Check sheet for the modelled part. Datum: model origin and axes. Units: mm. Face numbers are marked on the shaded views. A direction names the side the tool comes from. Give positions to 0.01 mm unless a question says otherwise; leave off trailing zeros. Order: outer loops, then holes, each group sorted by start corner. A loop starts at its lowest first (then second) coordinate and runs counter-clockwise, first axis right, second up.
```python
from build123d import *
from OCP.BRepFilletAPI import BRepFilletAPI_MakeChamfer

# Parameters (mm, degrees)
SKETCH1_W                                       = 42.2
SKETCH1_H                                       = 42.2
SKETCH1_R                                       = 12.5
SKETCH1_R_2                                     = 2
BOSS_EXTRUDE1_DEPTH                             = 2
SKETCH2_W                                       = 42.2
SKETCH2_H                                       = 20
SKETCH2_R                                       = 1.625
BOSS_EXTRUDE2_DEPTH                             = 5
BOSS_EXTRUDE3_DEPTH                             = 3.5
BOSS_EXTRUDE3_DEPTH_BACK                        = 2
SKETCH3_W                                       = 8.75
SKETCH3_H                                       = 23.25
SKETCH3_W_2                                     = 2.5
SKETCH3_H_2                                     = 7
CUT_EXTRUDE1_START                              = -3.5
SKETCH4_W                                       = 4.5
SKETCH4_H                                       = 7
CUT_EXTRUDE1_DEPTH                              = 3.5
CSK_FOR_M3_FLAT_HEAD_MACHINE_SCREW1_D           = 3.4
CSK_FOR_M3_FLAT_HEAD_MACHINE_SCREW1_CSINK_D     = 6.5
CSK_FOR_M3_FLAT_HEAD_MACHINE_SCREW1_CSINK_ANGLE = 90
SKETCH10_W                                      = 8.75
SKETCH10_H                                      = 23.25
SKETCH10_W_2                                    = 2.5
SKETCH10_H_2                                    = 7
BOSS_EXTRUDE4_DEPTH                             = 4
CUT_EXTRUDE3_DEPTH                              = 10
CHAMFER1_SIZE                                   = 10
FILLET2_R                                       = 3
FILLET3_R                                       = 3
FILLET4_R                                       = 3
CHAMFER2_SIZE                                   = 1
CHAMFER2_SIZE2                                  = 0.707106781
CHAMFER3_SIZE                                   = 0.5


with BuildPart() as part:
    # Sketch1 → Boss-Extrude1 (new, symmetric)
    with BuildSketch(Plane.XY.offset(1.5)):
        Rectangle(SKETCH1_W, SKETCH1_H)
        Circle(SKETCH1_R, mode=Mode.SUBTRACT)
        with Locations((15.5, 15.5)):
            Circle(SKETCH1_R_2, mode=Mode.SUBTRACT)
        with Locations((15.5, -15.5)):
            Circle(SKETCH1_R_2, mode=Mode.SUBTRACT)
        with Locations((-15.5, -15.5)):
            Circle(SKETCH1_R_2, mode=Mode.SUBTRACT)
        with Locations((-15.5, 15.5)):
            Circle(SKETCH1_R_2, mode=Mode.SUBTRACT)
    extrude(amount=BOSS_EXTRUDE1_DEPTH, both=True)

    # Sketch2 → Boss-Extrude2 (add)
    with BuildSketch(Plane.XZ.offset(21.1)):
        Rectangle(SKETCH2_W, SKETCH2_H)
        with Locations(Location((8, 7.5, 0), (0, 0, 270))):
            Circle(SKETCH2_R, mode=Mode.SUBTRACT)
        with Locations(Location((8, -7.5, 0), (0, 0, 270))):
            Circle(SKETCH2_R, mode=Mode.SUBTRACT)
        with Locations(Location((-8, -7.5, 0), (0, 0, 270))):
            Circle(SKETCH2_R, mode=Mode.SUBTRACT)
        with Locations(Location((-8, 7.5, 0), (0, 0, 270))):
            Circle(SKETCH2_R, mode=Mode.SUBTRACT)
    extrude(amount=BOSS_EXTRUDE2_DEPTH)

    # Sketch3 → Boss-Extrude3 (add, two sides: drawn at the far end of the back side and taken through both)
    # profile 1 of 2: a face of its own
    with BuildSketch(Plane.XY.offset(-BOSS_EXTRUDE3_DEPTH_BACK)):
        with Locations((-25.475, -14.475)):
            Rectangle(SKETCH3_W, SKETCH3_H)
        with Locations((-24.1, -9.1)):
            Rectangle(SKETCH3_W_2, SKETCH3_H_2, mode=Mode.SUBTRACT)
        with Locations((-24.1, -19.85)):
            Rectangle(SKETCH3_W_2, SKETCH3_H_2, mode=Mode.SUBTRACT)
    # profile 2 of 2: a face of its own
    with BuildSketch(Plane.XY.offset(-BOSS_EXTRUDE3_DEPTH_BACK)):
        with Locations((25.475, -14.475)):
            Rectangle(SKETCH3_W, SKETCH3_H)
        with Locations((24.1, -9.1)):
            Rectangle(SKETCH3_W_2, SKETCH3_H_2, mode=Mode.SUBTRACT)
        with Locations((24.1, -19.85)):
            Rectangle(SKETCH3_W_2, SKETCH3_H_2, mode=Mode.SUBTRACT)
    extrude(amount=BOSS_EXTRUDE3_DEPTH + BOSS_EXTRUDE3_DEPTH_BACK)

    # Sketch4 → Cut-Extrude1 (cut)
    with BuildSketch(Plane.XY.offset(3.5).offset(CUT_EXTRUDE1_START)):
        with Locations((-27.6, -9.1)):
            Rectangle(SKETCH4_W, SKETCH4_H)
        with Locations((-27.6, -19.85)):
            Rectangle(SKETCH4_W, SKETCH4_H)
        with Locations((27.6, -19.85)):
            Rectangle(SKETCH4_W, SKETCH4_H)
        with Locations((27.6, -9.1)):
            Rectangle(SKETCH4_W, SKETCH4_H)
    extrude(amount=CUT_EXTRUDE1_DEPTH, mode=Mode.SUBTRACT)

    # CSK for M3 Flat Head Machine Screw1 (through all)
    with Locations(Plane(origin=(0, -21.1, 0), x_dir=(1, 0, 0), z_dir=(0, 1, 0))):
        with Locations((-8, -7.5), (8, -7.5), (-8, 7.5), (8, 7.5)):
            CounterSinkHole(CSK_FOR_M3_FLAT_HEAD_MACHINE_SCREW1_D / 2, CSK_FOR_M3_FLAT_HEAD_MACHINE_SCREW1_CSINK_D / 2, counter_sink_angle=CSK_FOR_M3_FLAT_HEAD_MACHINE_SCREW1_CSINK_ANGLE)

    # Sketch10 → Boss-Extrude4 (add)
    # profile 1 of 2: a face of its own
    with BuildSketch(Plane(origin=(0, 0, -0.5), x_dir=(-1, 0, 0), z_dir=(0, 0, -1))):
        with Locations((25.475, -14.475)):
            Rectangle(SKETCH10_W, SKETCH10_H)
        with Locations((24.1, -19.85)):
            Rectangle(SKETCH10_W_2, SKETCH10_H_2, mode=Mode.SUBTRACT)
        with Locations((24.1, -9.1)):
            Rectangle(SKETCH10_W_2, SKETCH10_H_2, mode=Mode.SUBTRACT)
    # profile 2 of 2: a face of its own
    with BuildSketch(Plane(origin=(0, 0, -0.5), x_dir=(-1, 0, 0), z_dir=(0, 0, -1))):
        with Locations((-25.475, -14.475)):
            Rectangle(SKETCH10_W, SKETCH10_H)
        with Locations((-24.1, -19.85)):
            Rectangle(SKETCH10_W_2, SKETCH10_H_2, mode=Mode.SUBTRACT)
        with Locations((-24.1, -9.1)):
            Rectangle(SKETCH10_W_2, SKETCH10_H_2, mode=Mode.SUBTRACT)
    extrude(amount=BOSS_EXTRUDE4_DEPTH)

    # Sketch11 → Cut-Extrude3 (cut)
    with BuildSketch(Plane(origin=(0, -21.1, 0), x_dir=(1, 0, 0), z_dir=(0, 1, 0))):
        Polygon((-21.1, -3.5), (-15.1, -10), (-21.1, -10), align=None)
        Polygon((15.1, -10), (21.1, -10), (21.1, -3.5), align=None)
        Polygon((-21.1, 10), (-21.1, 4.5), (-15.1, 10), align=None)
        Polygon((21.1, 4.5), (21.1, 10), (15.1, 10), align=None)
    extrude(amount=-CUT_EXTRUDE3_DEPTH, mode=Mode.SUBTRACT)

    # Chamfer1
    # the kernel refuses this chamfer: 10 mm, written as the material it adds along each edge
    with BuildSketch(Plane(origin=(-21.1, -2.85, 3.5), x_dir=(0.027495876610585973, 0.9996219169112968, 0), z_dir=(0, 0, -1))) as chamfer1_piece_1_section:
        Polygon((CHAMFER1_SIZE * 0.999621916911, -CHAMFER1_SIZE * 0.0274958766106), (-CHAMFER1_SIZE * 0.0274958766106, -CHAMFER1_SIZE * 0.999621916911), (0, 0), align=None)
    chamfer1_piece_1 = extrude(amount=4, mode=Mode.PRIVATE)
    chamfer1_piece_1 = split(chamfer1_piece_1, bisect_by=Plane(origin=(-21.1, 0.400261982, 1.5), z_dir=(-1, 0, 0)), keep=Keep.TOP, mode=Mode.PRIVATE)
    chamfer1_piece_1 = split(chamfer1_piece_1, bisect_by=Plane(origin=(-29.85, 0.400261982, 1.5), z_dir=(1, 0, 0)), keep=Keep.TOP, mode=Mode.PRIVATE)
    add(chamfer1_piece_1)
    with BuildSketch(Plane(origin=(-21.1, -2.85, 3.5), x_dir=(0.027495876610585973, 0.9996219169112968, 0), z_dir=(0, 0, -1))) as chamfer1_piece_2_section:
        Polygon((CHAMFER1_SIZE * 0.999621916911, -CHAMFER1_SIZE * 0.0274958766106), (-CHAMFER1_SIZE * 0.0274958766106, -CHAMFER1_SIZE * 0.999621916911), (0, 0), align=None)
    chamfer1_piece_2 = extrude(amount=29.71682988, mode=Mode.PRIVATE)
    chamfer1_piece_2 = split(chamfer1_piece_2, bisect_by=Plane(origin=(-24.403786138, 0.400261982, -0.5), z_dir=(0, 0, -1)), keep=Keep.TOP, mode=Mode.PRIVATE)
    chamfer1_piece_2 = split(chamfer1_piece_2, bisect_by=Plane(origin=(-21.1, 0.400261982, -2.5), z_dir=(-1, 0, 0)), keep=Keep.TOP, mode=Mode.PRIVATE)
    chamfer1_piece_2 = split(chamfer1_piece_2, bisect_by=Plane(origin=(-24.403786138, 0.400261982, -4.5), z_dir=(0, 0, 1)), keep=Keep.TOP, mode=Mode.PRIVATE)
    chamfer1_piece_2 = split(chamfer1_piece_2, bisect_by=Plane(origin=(-29.85, 0.400261982, -2.5), z_dir=(1, 0, 0)), keep=Keep.TOP, mode=Mode.PRIVATE)
    add(chamfer1_piece_2)
    with BuildSketch(Plane(origin=(21.1, -2.85, 3.5), x_dir=(-0.027495876610585973, 0.9996219169112968, 0), z_dir=(0, 0, -1))) as chamfer1_piece_3_section:
        Polygon((CHAMFER1_SIZE * 0.999621916911, CHAMFER1_SIZE * 0.0274958766106), (-CHAMFER1_SIZE * 0.0274958766106, CHAMFER1_SIZE * 0.999621916911), (0, 0), align=None)
    chamfer1_piece_3 = extrude(amount=4, mode=Mode.PRIVATE)
    chamfer1_piece_3 = split(chamfer1_piece_3, bisect_by=Plane(origin=(21.1, 0.400261982, 1.5), z_dir=(1, 0, 0)), keep=Keep.TOP, mode=Mode.PRIVATE)
    chamfer1_piece_3 = split(chamfer1_piece_3, bisect_by=Plane(origin=(29.85, 0.400261982, 1.5), z_dir=(-1, 0, 0)), keep=Keep.TOP, mode=Mode.PRIVATE)
    add(chamfer1_piece_3)
    with BuildSketch(Plane(origin=(21.1, -2.85, 3.5), x_dir=(-0.027495876610585973, 0.9996219169112968, 0), z_dir=(0, 0, -1))) as chamfer1_piece_4_section:
        Polygon((CHAMFER1_SIZE * 0.999621916911, CHAMFER1_SIZE * 0.0274958766106), (-CHAMFER1_SIZE * 0.0274958766106, CHAMFER1_SIZE * 0.999621916911), (0, 0), align=None)
    chamfer1_piece_4 = extrude(amount=29.71682988, mode=Mode.PRIVATE)
    chamfer1_piece_4 = split(chamfer1_piece_4, bisect_by=Plane(origin=(24.403786138, 0.400261982, -0.5), z_dir=(0, 0, -1)), keep=Keep.TOP, mode=Mode.PRIVATE)
    chamfer1_piece_4 = split(chamfer1_piece_4, bisect_by=Plane(origin=(21.1, 0.400261982, -2.5), z_dir=(1, 0, 0)), keep=Keep.TOP, mode=Mode.PRIVATE)
    chamfer1_piece_4 = split(chamfer1_piece_4, bisect_by=Plane(origin=(24.403786138, 0.400261982, -4.5), z_dir=(0, 0, 1)), keep=Keep.TOP, mode=Mode.PRIVATE)
    chamfer1_piece_4 = split(chamfer1_piece_4, bisect_by=Plane(origin=(29.85, 0.400261982, -2.5), z_dir=(-1, 0, 0)), keep=Keep.TOP, mode=Mode.PRIVATE)
    add(chamfer1_piece_4)

    # Fillet2
    fillet2_edges = [part.edges().sort_by_distance(p)[0] for p in [
        (21.1, 7.15, 1.5),
        (-21.1, 7.15, 1.5),
        (29.85, -1.6, -0.5),
        (-29.85, -1.6, -0.5),
    ]]
    fillet(fillet2_edges, radius=FILLET2_R)

    # Fillet3
    fillet3_edges = [part.edges().sort_by_distance(p)[0] for p in [
        (-21.1, 21.1, 1.5),
        (21.1, 21.1, 1.5),
    ]]
    fillet(fillet3_edges, radius=FILLET3_R)

    # Fillet4
    fillet4_edges = [part.edges().sort_by_distance(p)[0] for p in [
        (21.1, -23.6, -4.5),
        (-21.1, -23.6, -4.5),
        (-15.1, -23.6, 10),
        (15.1, -23.6, 10),
        (-15.1, -23.6, -10),
        (15.1, -23.6, -10),
        (-21.1, -23.6, 3.5),
        (21.1, -23.6, 3.5),
    ]]
    fillet(fillet4_edges, radius=FILLET4_R)

    # Chamfer2: one chamfer whose edges measure the first distance from different faces: ONE call of the kernel's chamfer builder (chamfer() names one face for all edges)
    chamfer2_edges_1 = [part.edges().sort_by_distance(p)[0] for p in [
        (21.1, 7.15, -2.5),
    ]]
    chamfer2_side_1 = [part.faces().sort_by_distance(p)[0] for p in [
        (25.242344349, 3.007655651, -0.618229543),
    ]]
    chamfer2_edges_2 = [part.edges().sort_by_distance(p)[0] for p in [
        (-21.1, 7.15, -2.5),
    ]]
    chamfer2_side_2 = [part.faces().sort_by_distance(p)[0] for p in [
        (-25.242344349, 3.007655651, -0.618229543),
    ]]
    chamfer2 = BRepFilletAPI_MakeChamfer(part.part.solid().wrapped)
    for e in chamfer2_edges_1:
        chamfer2.Add(CHAMFER2_SIZE, CHAMFER2_SIZE2, e.wrapped, chamfer2_side_1[0].wrapped)  # the first distance lies on this face
    for e in chamfer2_edges_2:
        chamfer2.Add(CHAMFER2_SIZE, CHAMFER2_SIZE2, e.wrapped, chamfer2_side_2[0].wrapped)  # the first distance lies on this face
    add(Compound.cast(chamfer2.Shape()), mode=Mode.REPLACE)

    # Chamfer3
    chamfer3_edges = [part.edges().sort_by_distance(p)[0] for p in [
        (25.35, -9.1, 0),
        (25.35, -19.85, 0),
        (-25.35, -19.85, 0),
        (-25.35, -9.1, 0),
    ]]
    chamfer(chamfer3_edges, length=CHAMFER3_SIZE)


solid = part.part
```
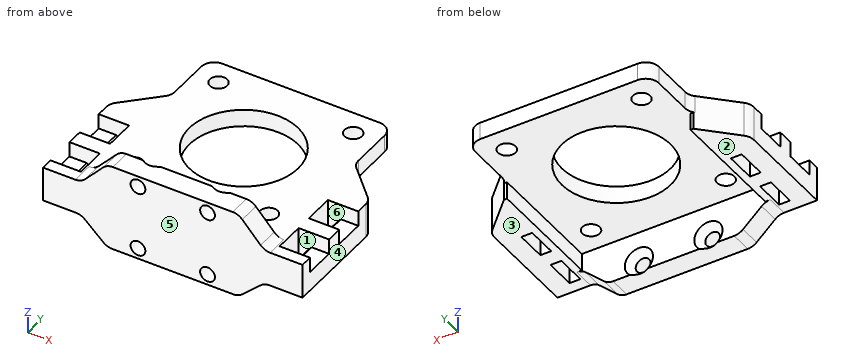
(1) Cross-section at B-B on y = 0. Enter the section's corners in (x, z).
Response values:
outline: (-28.25, -4.5) - (-21.1, -4.5) - (-21.1, -0.5) - (-12.5, -0.5) - (-12.5, 3.5) - (-28.25, 3.5) - close; (12.5, -0.5) - (21.1, -0.5) - (21.1, -4.5) - (28.25, -4.5) - (28.25, 3.5) - (12.5, 3.5) - close
(2) Cross-section at C-C on x = 2.5. Enter the section's corners in (y, z).
Response values:
outline: (-26.1, -10) - (-21.1, -10) - (-21.1, -0.5) - (-12.25, -0.5) - (-12.25, 3.5) - (-21.1, 3.5) - (-21.1, 10) - (-26.1, 10) - close; (12.25, -0.5) - (21.1, -0.5) - (21.1, 3.5) - (12.25, 3.5) - close
(3) Cross-section at A-A on y = 15.5. Enter the section's corners in (x, z), then the cut area to 3 significant figures.
Response values:
outline: (-21.1, -0.5) - (-17.5, -0.5) - (-17.5, 3.5) - (-21.1, 3.5) - close; (-13.5, -0.5) - (13.5, -0.5) - (13.5, 3.5) - (-13.5, 3.5) - close; (17.5, -0.5) - (21.1, -0.5) - (21.1, 3.5) - (17.5, 3.5) - close
area: 137 mm2
(4) Material ranges on L1, parallel to Y at x = -15.5, z = 0.5; L2, parallel to X at y = -24.8, z = 7.5; L3, parallel to Y at x = 2.5, z = -3, recorded low to high.
Response values:
L1: y = -26.1 to -17.5, -13.5 to 13.5, 17.5 to 21.1
L2: x = -17.41 to -9.7, -6.3 to 6.3, 9.7 to 17.41
L3: y = -26.1 to -21.1
(5) Cross-section at D-D on z = -2. Enter the section's corners in (x, y), then the cut area to 3 significant figures.
Response values:
outline: (-29.85, -26.1) - (29.85, -26.1) - (29.85, -2.84) arc R3 ccw to (28.97, -0.72) - (21.81, 6.44) - (21.1, 6.44) - (21.1, -21.1) - (-21.1, -21.1) - (-21.1, 6.44) - (-21.81, 6.44) - (-28.97, -0.72) arc R3 ccw to (-29.85, -2.84) - close; hole (-25.35, -23.35) - (-22.85, -23.35) - (-22.85, -16.35) - (-25.35, -16.35) - close; hole (-25.35, -12.6) - (-22.85, -12.6) - (-22.85, -5.6) - (-25.35, -5.6) - close; hole (22.85, -23.35) - (25.35, -23.35) - (25.35, -16.35) - (22.85, -16.35) - close; hole (22.85, -12.6) - (25.35, -12.6) - (25.35, -5.6) - (22.85, -5.6) - close
area: 645 mm2
(6) Set-up check for the marked faces 1, 2 and 3: record each of +Z, -Z, +X, -X, +Y, -Y from which the full face is reachable in a straight line by a thin tool's end or side.
Response values:
face 1: +Z
face 2: -Z, -X, +Y
face 3: -Z, +X, +Y
(7) Release check for a two-part mould opening along Y. For the marked faces 4, 5 and 6 record: released by +Y, released by -Y, zero draft, split by the parting line, or undercut.
Response values:
face 4: zero draft
face 5: released by -Y
face 6: undercut
(8) Gauge pin test, flat ends, axial feed: pin 1 Ø5 at (x, y) = (5, 15) entering from -Z; pin 2 Ø0.8 at (x, z) = (21.5, -3) entering from +Y; pin 3 Ø6 at (y, z) = (-19, 7.5) entering from +X; pin 4 Ø2 at (y, z) = (-8.5, 0.5) entering from -X. Record the tip position at first contact, or that the pin passes through.
Response values:
pin 1: stops at z = -0.5
pin 2: stops at y = 6.44
pin 3: stops at x = 19.39
pin 4: stops at x = -29.85
